Source: CAD feature listing. Evaluate the final solid. Frame: model axes, mm. A direction names the side the tool comes from. Coordinates: 2 decimals unless noted, no trailing zeros. Write each loop counter-clockwise with the first axis right and the second up, starting at its lowest first coordinate (ties: lowest second). Pieces come first, ordered by that corner, then holes. Notation, with made-up numbers: (-39.75, 62) -> (1.25, 62) arc R18 ccw to (1.25, 68) -> close; hole circle Ø11 at (14, -7.75). An arc over 180 degrees is marked (long way). One line per item, written item: value. Start each with the question number.
1. Section query A-A, the plane y = -39. Output: boundary loops of the cut face in (x, z).
2. First-contact query: P1, Ø1.1, axis at y = 0, z = 4, coming from the +X side; P2, Ø3, axis at x = 32, y = -39, coming from the +Z side. Flat tips, straight axial feed; report the tip coordinate or a pass-through.
3. Mould query, pull axis X, two halves, no side actions, for faces 1 (the flat face through (42, -1, 3)), 2 (the cylindrical face through (30.245, -37.391, 6.923)), 3 (the flat face through (-1, 1, 8)), 4 (the cylindrical face through (-33.126, -39.467, 2.867)). Classes: released by +X, released by -X, zero draft, split by the parting line, or undercut.
4. Access query for faces 5 (the flat face through (-1, 42, 4)), 6 (the cylindrical face through (-33.755, -37.391, 6.923)). Directions: +Z, -Z, +X, -X, +Y, -Y. A direction counts if a zero-diameter tool reaches every point of the face in a straight line with its end or side. Return the directions, or none.
5. Line query: line 1 (X direction, y = 33.5, z = 4); line 2 (Y direction, x = -32, z = 7). Output: solid intervals per line, ascending.
from build123d import *

# Parameters (mm, degrees)
SKETCH1_W                                      = 84
SKETCH1_H                                      = 84
BOSS_EXTRUDE1_DEPTH                            = 8
CBORE_FOR_2_SOCKET_HEAD_CAP_SCREW1_D           = 2.4384
CBORE_FOR_2_SOCKET_HEAD_CAP_SCREW1_DEPTH       = 8
CBORE_FOR_2_SOCKET_HEAD_CAP_SCREW1_CBORE_D     = 4.7625
CBORE_FOR_2_SOCKET_HEAD_CAP_SCREW1_CBORE_DEPTH = 2.1844
F_2_56_TAPPED_HOLE1_D                          = 1.778
F_2_56_TAPPED_HOLE1_DEPTH                      = 12
F_2_56_TAPPED_HOLE1_TIP                        = 0.53416509
F_2_56_TAPPED_HOLE2_D                          = 1.778
F_2_56_TAPPED_HOLE2_DEPTH                      = 12
F_2_56_TAPPED_HOLE2_TIP                        = 0.53416509
F_2_56_TAPPED_HOLE3_D                          = 1.778
F_2_56_TAPPED_HOLE3_DEPTH                      = 12
F_2_56_TAPPED_HOLE3_TIP                        = 0.53416509


with BuildPart() as part:
    # Sketch1 → Boss-Extrude1 (new body)
    with BuildSketch(Plane.XY):
        Rectangle(SKETCH1_W, SKETCH1_H)
    extrude(amount=BOSS_EXTRUDE1_DEPTH)

    # CBORE for #2 Socket Head Cap Screw1
    with Locations(Plane(origin=(-32, -39, 8), x_dir=(1, 0, 0), z_dir=(0, 0, 1))):
        with Locations((0, 0), (64, 0)):
            CounterBoreHole(CBORE_FOR_2_SOCKET_HEAD_CAP_SCREW1_D / 2, CBORE_FOR_2_SOCKET_HEAD_CAP_SCREW1_CBORE_D / 2, CBORE_FOR_2_SOCKET_HEAD_CAP_SCREW1_CBORE_DEPTH, depth=CBORE_FOR_2_SOCKET_HEAD_CAP_SCREW1_DEPTH)

    # #2-56 Tapped Hole1
    with Locations(Plane(origin=(42, 0, 4), x_dir=(0, 0, 1), z_dir=(1, 0, 0))):
        with Locations((0, 0)):
            Hole(F_2_56_TAPPED_HOLE1_D / 2, depth=F_2_56_TAPPED_HOLE1_DEPTH)
            with Locations((0, 0, -(F_2_56_TAPPED_HOLE1_DEPTH + F_2_56_TAPPED_HOLE1_TIP / 2))):  # 118° drill point
                Cone(0, F_2_56_TAPPED_HOLE1_D / 2, F_2_56_TAPPED_HOLE1_TIP, mode=Mode.SUBTRACT)

    # #2-56 Tapped Hole2
    with Locations(Plane(origin=(-42, 0, 4), x_dir=(0, 0, -1), z_dir=(-1, 0, 0))):
        with Locations((0, 0)):
            Hole(F_2_56_TAPPED_HOLE2_D / 2, depth=F_2_56_TAPPED_HOLE2_DEPTH)
            with Locations((0, 0, -(F_2_56_TAPPED_HOLE2_DEPTH + F_2_56_TAPPED_HOLE2_TIP / 2))):  # 118° drill point
                Cone(0, F_2_56_TAPPED_HOLE2_D / 2, F_2_56_TAPPED_HOLE2_TIP, mode=Mode.SUBTRACT)

    # #2-56 Tapped Hole3
    with Locations(Plane(origin=(-32, 42, 4), x_dir=(0, 0, 1), z_dir=(0, 1, 0))):
        with Locations((0, 0), (0, 64)):
            Hole(F_2_56_TAPPED_HOLE3_D / 2, depth=F_2_56_TAPPED_HOLE3_DEPTH)
            with Locations((0, 0, -(F_2_56_TAPPED_HOLE3_DEPTH + F_2_56_TAPPED_HOLE3_TIP / 2))):  # 118° drill point
                Cone(0, F_2_56_TAPPED_HOLE3_D / 2, F_2_56_TAPPED_HOLE3_TIP, mode=Mode.SUBTRACT)


solid = part.part
Computed values:
1. outline: (-42, 0) -> (-33.22, 0) -> (-33.22, 5.82) -> (-34.38, 5.82) -> (-34.38, 8) -> (-42, 8) -> close; (-30.78, 0) -> (30.78, 0) -> (30.78, 5.82) -> (29.62, 5.82) -> (29.62, 8) -> (-29.62, 8) -> (-29.62, 5.82) -> (-30.78, 5.82) -> close; (33.22, 0) -> (42, 0) -> (42, 8) -> (34.38, 8) -> (34.38, 5.82) -> (33.22, 5.82) -> close
2. P1: stops at x = 29.8
2. P2: stops at z = 5.82
3. face 1: released by +X
3. face 2: undercut
3. face 3: zero draft
3. face 4: undercut
4. face 5: +Z, -Z, +X, -X, +Y
4. face 6: +Z
5. line 1: x = -42 to -32.89, -31.11 to 31.11, 32.89 to 42
5. line 2: y = -42 to -41.38, -36.62 to 42
